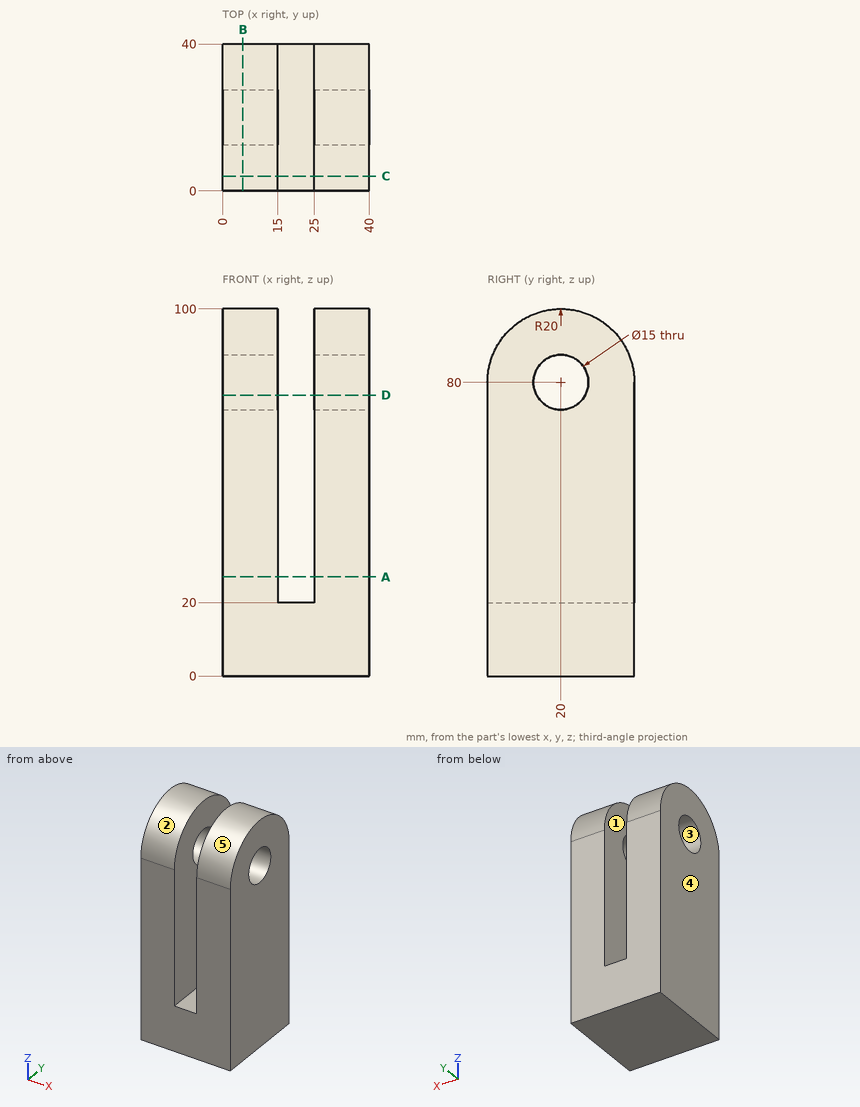
Geometry: see drawing. Coordinates: mm, zero at the bounding-box minimum. A direction names the side the tool comes from. Coordinates: 2 decimals unless noted, no trailing zeros. Order: outer loops, then holes, each group sorted by start corner. A loop starts at its lowest first (then second) coordinate and runs counter-clockwise, first axis right, second up. Notation, with made-up numbers: (14, 6) -> (71, 6) arc R3 ccw to (71, 11) -> close; hole circle Ø5 at (-15.75, -10.75). An arc over 180 degrees is marked (long way). Write each question's results on one line, items separated by ' | '. Start each with the question number.
1) Mould query, pull axis Z, two halves, no side actions, for the marked faces 3, 4 and 5. Classes: released by +Z, released by -Z, zero draft, split by the parting line, or undercut.
2) Set-up query: the marked faces 1 and 2. Return all of +Z, -Z, +X, -X, +Y, -Y with unobstructed straight access to the full face (end or side cutting, diameter ignored); none if empty.
3) Cut plane C-C, the plane y = 4. Output: boundary loops of the cut face in (x, z), and give its area (3 significant figures).
4) Material intervals for line 1 along X through (y, z) = (35, 56.5); line 2 along Z through (x, y) = (11, 20); line 3 along Y through (x, z) = (6, 80), sorted ascending.
5) Cut plane A-A, the plane z = 27. Output: boundary loops of the cut face in (x, y).
6) Cut plane D-D, the plane z = 76.5. Output: boundary loops of the cut face in (x, y), and give its area (3 significant figures).
7) First-contact query: pin 1 (3 mm diameter, centred on x = 18, y = 22, fed in from +Z); pin 2 (4 mm diameter, centred on x = 12, y = 12, fed in from +Z); pin 3 (5 mm diameter, centred on x = 25, y = 27.5, fed in from +Z). Flat tips, straight axial feed; report the tip coordinate or a pass-through.
8) Cut plane B-B, the plane x = 5.5. Output: boundary loops of the cut face in (y, z), and give its area (3 significant figures).
Checks:
1) face 3: undercut | face 4: zero draft | face 5: released by +Z
2) face 1: +Z, +Y, -Y | face 2: +Z, +X, -X
3) outline: (0, 0) -> (40, 0) -> (40, 92) -> (25, 92) -> (25, 20) -> (15, 20) -> (15, 92) -> (0, 92) -> close | area: 2,960 mm^2
4) line 1: 0 to 15, 25 to 40 | line 2: 0 to 72.5, 87.5 to 100 | line 3: 0 to 12.5, 27.5 to 40
5) outline: (0, 0) -> (15, 0) -> (15, 40) -> (0, 40) -> close; (25, 0) -> (40, 0) -> (40, 40) -> (25, 40) -> close
6) outline: (0, 0) -> (15, 0) -> (15, 13.37) -> (0, 13.37) -> close; (0, 26.63) -> (15, 26.63) -> (15, 40) -> (0, 40) -> close; (25, 0) -> (40, 0) -> (40, 13.37) -> (25, 13.37) -> close; (25, 26.63) -> (40, 26.63) -> (40, 40) -> (25, 40) -> close | area: 802 mm^2
7) pin 1: z = 20 | pin 2: z = 99.08 | pin 3: z = 99.36
8) outline: (0, 0) -> (40, 0) -> (40, 80) arc R20 ccw to (0, 80) -> close; hole circle Ø15 at (20, 80) | area: 3,650 mm^2
